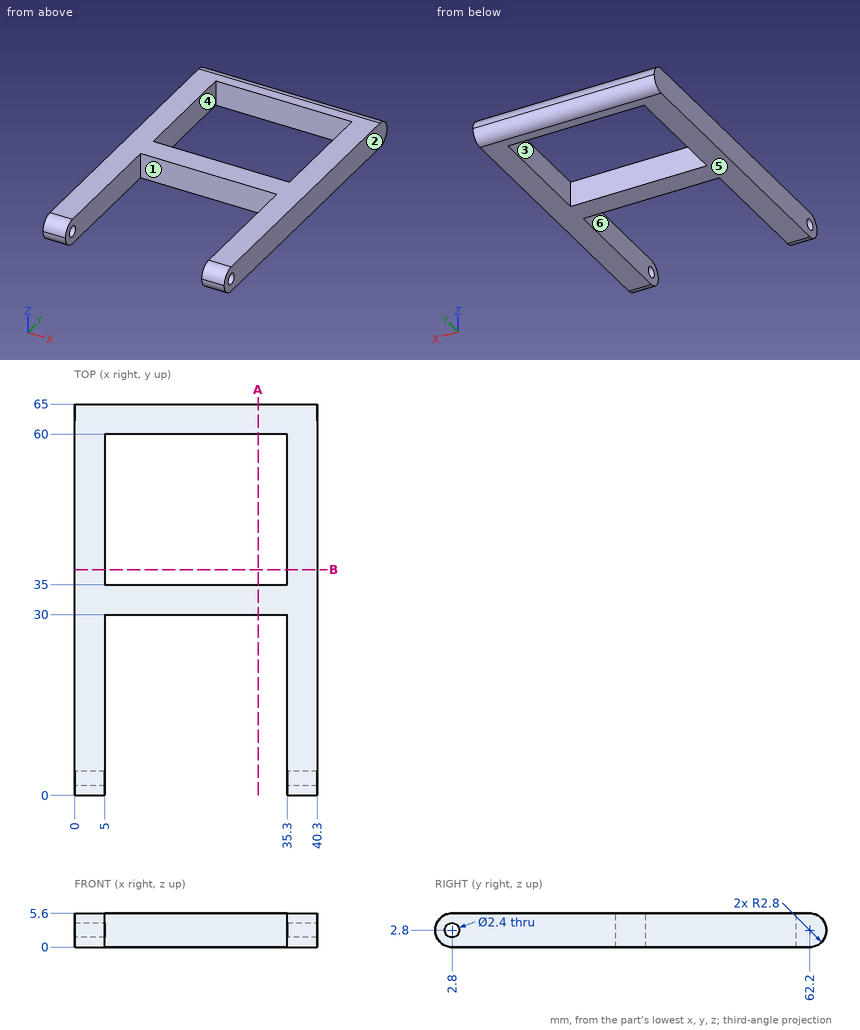
Input: dimensioned drawing with shaded views. Units: mm. Origin: part minimum x, y, z. A direction names the side the tool comes from. Coordinates: 2 decimals unless noted, no trailing zeros. Loops run counter-clockwise (first coordinate to the right, second up) from the corner with the lowest first, then second, coordinate; pieces in that order, holes last. Notation, with made-up numbers: (-11, 67) -> (6, 67) arc R25 ccw to (6, 103) -> close; hole circle Ø2 at (38, 50.25). An arc over 180 degrees is marked (long way). Use a Markdown table: item, result. Add a question column.
(1) Section query B-B, the plane y = 37.5. Return loops of the section in (x, z), plus the area to 3 significant figures.
(2) Access query for the marked faces 4, 5 and 6. Directions: +Z, -Z, +X, -X, +Y, -Y. A direction counts if a zero-diameter tool reaches every point of the face in a straight line with its end or side. Return the directions, or none.
(3) Mould query, pull axis Y, two halves, no side actions, for the marked faces 1, 2 and 3. Classes: pulls with the +Y half, pulls with the -Y half, needs draft (parallel to the pull), parting line crosses it, or undercut.
(4) Line query: line 1 along X through (y, z) = (56.5, 3.7); line 2 along Y through (x, z) = (15, 4.25); line 3 along Y through (x, z) = (32.5, 5.3). Output: solid intervals per line, ascending.
(5) Section query A-A, the plane x = 30.5. Return loops of the section in (y, z), plus the area to 3 significant figures.
(6) Pin query (flat end, axial travel): pin 1 Ø1.7 at (x, z) = (24.5, 3.5) entering from -Y; pin 2 Ø1 at (x, z) = (4.5, 1) entering from -Y; pin 3 Ø8 at (x, y) = (10, 37.5) entering from +Z. Return the tip coordinate at first contact, or that it passes through.
Answer:
| question | item | result |
|---|---|---|
| 1 | outline | (0, 0) -> (5, 0) -> (5, 5.6) -> (0, 5.6) -> close; (35.3, 0) -> (40.3, 0) -> (40.3, 5.6) -> (35.3, 5.6) -> close |
| 1 | area | 56.0 mm^2 |
| 2 | face 4 | +Z, -Z |
| 2 | face 5 | -Z, +X, -X, +Y, -Y |
| 2 | face 6 | +Z, -Z, -Y |
| 3 | face 1 | pulls with the -Y half |
| 3 | face 2 | needs draft |
| 3 | face 3 | undercut |
| 4 | line 1 | x = 0 to 5, 35.3 to 40.3 |
| 4 | line 2 | y = 30 to 35, 60 to 64.6 |
| 4 | line 3 | y = 30 to 35, 60 to 63.46 |
| 5 | outline | (30, 0) -> (35, 0) -> (35, 5.6) -> (30, 5.6) -> close; (60, 0) -> (62.2, 0) arc R2.8 ccw to (62.2, 5.6) -> (60, 5.6) -> close |
| 5 | area | 52.6 mm^2 |
| 6 | pin 1 | stops at y = 30 |
| 6 | pin 2 | stops at y = 0.32 |
| 6 | pin 3 | stops at z = 5.6 |
